Read the model definition and answer for the solid it produces. Units are mm, in the model's axes. Round coordinates to 2 decimals unless told otherwise and drop trailing zeros. Order: outer loops, then holes, each group sorted by start corner. A loop starts at its lowest first (then second) coordinate and runs counter-clockwise, first axis right, second up. Notation, with made-up numbers: (13, -28.5) -> (46, -28.5) arc R22 ccw to (46, 1.5) -> close; hole circle Ø4 at (35, -0.5). An arc over 180 degrees is marked (long way). One line per item, written item: value. Start each with the question number.
1. Section C-C (x = 31.5) is taken. Give the vertices of the cut face in (y, z).
2. Flat-ended cylindrical pins translate along their axes: pin 1 Ø3 at (y, z) = (-66.5, 15.5) entering from +X; pin 2 Ø1 at (y, z) = (15.5, 84.5) entering from -X; pin 3 Ø12 at (y, z) = (43.5, 203) entering from +X. Find the tip coordinate at first contact, or state that the pin passes through.
3. Consider line 1 (X direction, y = -58, z = 40.5); line 2 (X direction, y = 19.5, z = -199); line 3 (Y direction, x = -16.5, z = -134.5). Determine where each line is inside the solid, lowest interval first.
4. Section A-A (z = -32.5) is taken. Give the vertices of the cut face in (x, y).
5. Section B-B (y = -69) is taken. Give the vertices of the cut face in (x, z).
from build123d import *

# Parameters (mm, degrees)
FUSELAGE_START     = -254
FUSELAGE_OUTLINE_R = 139.7
FUSELAGE_DEPTH     = 508


# Read off the part's stored shape, not the designer's step: FuseLage
with BuildPart() as part:
    # FuseLage outline → FuseLage (new body)
    with BuildSketch(Plane.XY.offset(FUSELAGE_START)):
        Circle(FUSELAGE_OUTLINE_R)
    extrude(amount=FUSELAGE_DEPTH)


solid = part.part
Answer:
1. outline: (-136.1, -254) -> (136.1, -254) -> (136.1, 254) -> (-136.1, 254) -> close
2. pin 1: x = 123.66
2. pin 2: x = -138.89
2. pin 3: x = 134.57
3. line 1: -127.09 to 127.09
3. line 2: -138.33 to 138.33
3. line 3: -138.72 to 138.72
4. outline: circle Ø279.4 at (0, 0)
5. outline: (-121.47, -254) -> (121.47, -254) -> (121.47, 254) -> (-121.47, 254) -> close
